```python
from build123d import *

# Parameters (mm, degrees)
SKETCH1_W           = 32
SKETCH1_H           = 32
SKETCH1_R           = 3.5
BOSS_EXTRUDE1_DEPTH = 7
CHAMFER2_SIZE       = 2
CHAMFER2_SIZE2      = 1.154700538


with BuildPart() as part:
    # Sketch1 → Boss-Extrude1 (new body)
    with BuildSketch(Plane(origin=(0, 0, 0), x_dir=(1, 0, 0), z_dir=(0, 1, 0))):
        Rectangle(SKETCH1_W, SKETCH1_H)
        with Locations(Location((-8, 0, 0), (0, 0, 270))):
            Circle(SKETCH1_R, mode=Mode.SUBTRACT)
        with Locations(Location((8, 0, 0), (0, 0, 270))):
            Circle(SKETCH1_R, mode=Mode.SUBTRACT)
    extrude(amount=BOSS_EXTRUDE1_DEPTH)

    # Chamfer2
    chamfer2_edges = [part.edges().sort_by_distance(p)[0] for p in [
        (-8, 7, -3.5),
        (8, 7, -3.5),
    ]]
    chamfer2_side = [part.faces().sort_by_distance(p)[0] for p in [
        (0, 7, 0),
    ]]
    chamfer(chamfer2_edges, length=CHAMFER2_SIZE, length2=CHAMFER2_SIZE2, reference=chamfer2_side[0])


solid = part.part
```
Source: CAD feature listing. Evaluate the final solid. Frame: model axes, mm. Coordinates: 2 decimals unless noted, no trailing zeros. Loops run counter-clockwise (first coordinate to the right, second up) from the corner with the lowest first, then second, coordinate; pieces in that order, holes last. Notation, with made-up numbers: M 38.25,47.25 L 64.25,47.25 A23 cw 64.25,81.25 Z; hole C 89.25,-24.75 d5. An arc over 180 degrees is marked long. Use a Markdown table: item, result. Add a question column.
Q1. Material intervals for L1, parallel to X at y = 2.95, z = 0; L2, parallel to X at y = 1, z = -1.5; L3, parallel to Z at x = -9.5, y = 6.5, sorted ascending.
Q2. Section query B-B, the plane z = 0. Return loops of the section in (x, y), and give its area (3 significant figures).
Q3. First-contact query: pin 1 (4 mm diameter, centred on x = -8, z = 0, fed in from -Y); pin 2 (9 mm diameter, centred on x = 8, z = 0, fed in from +Y). Flat tips, straight axial feed; report the tip coordinate or a pass-through.
Q4. Section query A-A, the plane x = -8. Return loops of the section in (y, z).
Q5. Draft query along Z for faces 1 (the flat face through (0, 3, -16)), 2 (the flat face through (16, 3, 0)), 3 (the cylindrical face through (4.583, 2.882, -0.759)). Return one class per face: pulls with the +Z half, pulls with the -Z half, needs draft (parallel to the pull), parting line crosses it, or undercut.
Q6. Section query C-C, the plane y = 3.5. Return loops of the section in (x, z), and give its area (3 significant figures).
Result:
| question | item | result |
|---|---|---|
| 1 | L1 | x = -16 to -11.5, -4.5 to 4.5, 11.5 to 16 |
| 1 | L2 | x = -16 to -11.16, -4.84 to 4.84, 11.16 to 16 |
| 1 | L3 | z = -16 to -4.38, 4.38 to 16 |
| 2 | outline | M -16,0 L -11.5,0 L -11.5,5.85 L -13.5,7 L -16,7 Z; M -4.5,0 L 4.5,0 L 4.5,5.85 L 2.5,7 L -2.5,7 L -4.5,5.85 Z; M 11.5,0 L 16,0 L 16,7 L 13.5,7 L 11.5,5.85 Z |
| 2 | area | 121 mm2 |
| 3 | pin 1 | passes through |
| 3 | pin 2 | stops at y = 6.42 |
| 4 | outline | M 0,-16 L 7,-16 L 7,-5.5 L 5.85,-3.5 L 0,-3.5 Z; M 0,3.5 L 5.85,3.5 L 7,5.5 L 7,16 L 0,16 Z |
| 5 | face 1 | pulls with the -Z half |
| 5 | face 2 | needs draft |
| 5 | face 3 | undercut |
| 6 | outline | M -16,-16 L 16,-16 L 16,16 L -16,16 Z; hole C -8,0 d7; hole C 8,0 d7 |
| 6 | area | 947 mm2 |
